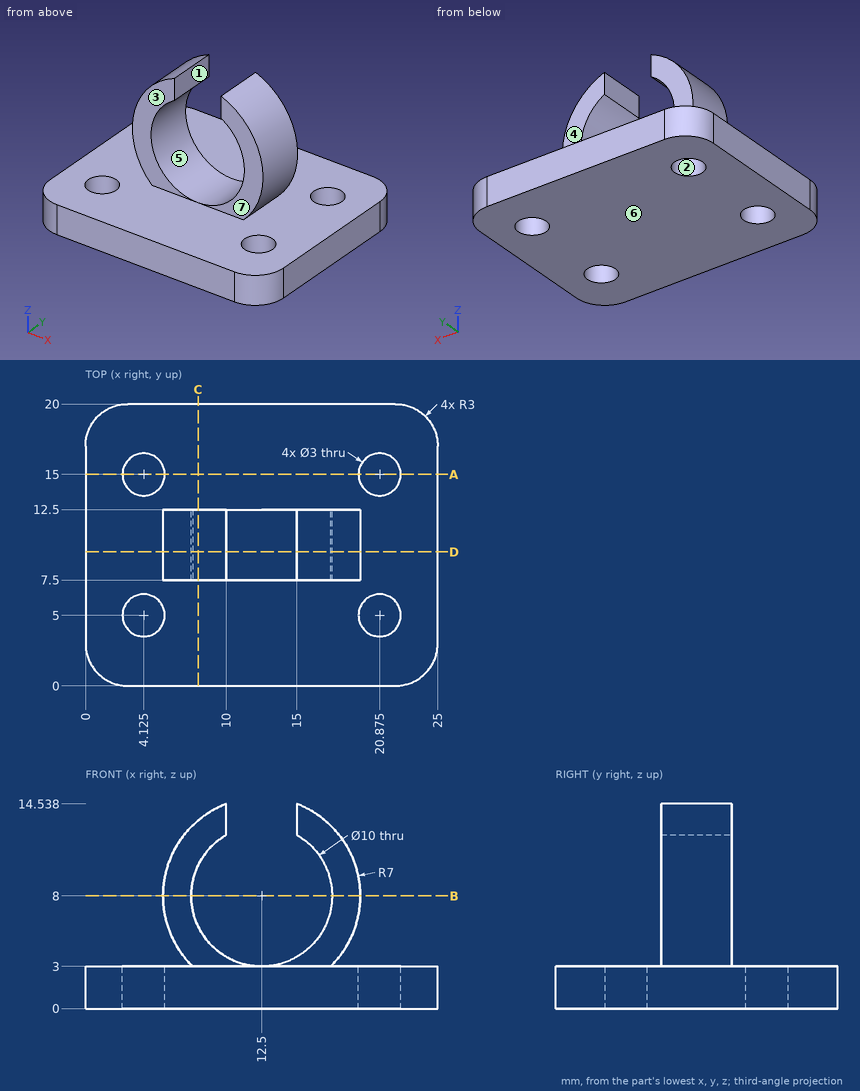
Print and shaded views of the part. All mm, measured from the part's lowest x, y and z. A direction names the side the tool comes from. Round coordinates to 2 decimals unless told otherwise and drop trailing zeros. Order: outer loops, then holes, each group sorted by start corner. A loop starts at its lowest first (then second) coordinate and runs counter-clockwise, first axis right, second up.
Q1. Drop flat-ended pins along their axis: pin 1 (5 mm diameter, centred on x = 20.875, y = 15, fed in from +Z); pin 2 (5 mm diameter, centred on x = 7, z = 9.5, fed in from +Y); pin 3 (1.8 mm diameter, centred on y = 9, z = 13, fed in from -X). Give the stop position or say it passes through.
Q2. Which spindle directions (+Z, -Z, +X, -X, +Y, -Y) get a long thin tool onto all of the face, cutting with end or side? Do the marked faces 1, 2, 3 and 4. Say none if no direction does.
Q3. Slice it at A-A (y = 15). Write the cut outline in (x, z) (1 decimal).
Q4. Two-plate mould, pull along Z, no slides. Class the marked faces 5, 6 and 7: pulls with the +Z half, pulls with the -Z half, needs draft (parallel to the pull), parting line crosses it, or undercut.
Q5. Wall check: L1, parallel to Y at x = 21, z = 1.5 (1 decimal); L2, parallel to X at y = 15, z = 2.3 (1 decimal); L3, parallel to Y at x = 17, z = 3.5. Give the ranges that are in metal, low to high.
Q6. Slice it at D-D (y = 9.5). Write the cut outline in (x, z).
Q7. Slice it at B-B (z = 8). Write the cut outline in (x, y), and give its area (3 significant figures).
Q8. Slice it at C-C (x = 8). Write the cut outline in (y, z).
Results below:
1. pin 1: stops at z = 3
1. pin 2: stops at y = 12.5
1. pin 3: stops at x = 6.83
2. face 1: +Z, +Y, -Y
2. face 2: +Z, -Z
2. face 3: +Z, +X, -X, -Y
2. face 4: +Z, +X, -X, +Y
3. outline: (0, 0) - (2.6, 0) - (2.6, 3) - (0, 3) - close; (5.6, 0) - (19.4, 0) - (19.4, 3) - (5.6, 3) - close; (22.4, 0) - (25, 0) - (25, 3) - (22.4, 3) - close
4. face 5: undercut
4. face 6: pulls with the -Z half
4. face 7: needs draft
5. L1: y = 0 to 3.5, 6.5 to 13.5, 16.5 to 20
5. L2: x = 0 to 2.6, 5.6 to 19.4, 22.4 to 25
5. L3: y = 7.5 to 12.5
6. outline: (0, 0) - (25, 0) - (25, 3) - (17.4, 3) arc R7 ccw to (15, 14.54) - (15, 12.33) arc R5 cw (long way) to (10, 12.33) - (10, 14.54) arc R7 ccw to (7.6, 3) - (0, 3) - close
7. outline: (5.5, 7.5) - (7.5, 7.5) - (7.5, 12.5) - (5.5, 12.5) - close; (17.5, 7.5) - (19.5, 7.5) - (19.5, 12.5) - (17.5, 12.5) - close
7. area: 20.0 mm2
8. outline: (0, 0) - (20, 0) - (20, 3) - (12.5, 3) - (12.5, 5.82) - (7.5, 5.82) - (7.5, 3) - (0, 3) - close; (7.5, 10.18) - (12.5, 10.18) - (12.5, 13.36) - (7.5, 13.36) - close
